Input: dimensioned drawing with shaded views. Units: mm. Origin: part minimum x, y, z. Round coordinates to 2 decimals unless told otherwise and drop trailing zeros. Order: outer loops, then holes, each group sorted by start corner. A loop starts at its lowest first (then second) coordinate and runs counter-clockwise, first axis right, second up. Notation, with made-up numbers: (86, 61) - (104, 61) arc R16 cw to (104, 92) - close; hole circle Ø9 at (72, 69.25). An arc over 180 degrees is marked (long way). One line per item, written item: value. Start each with the question number.
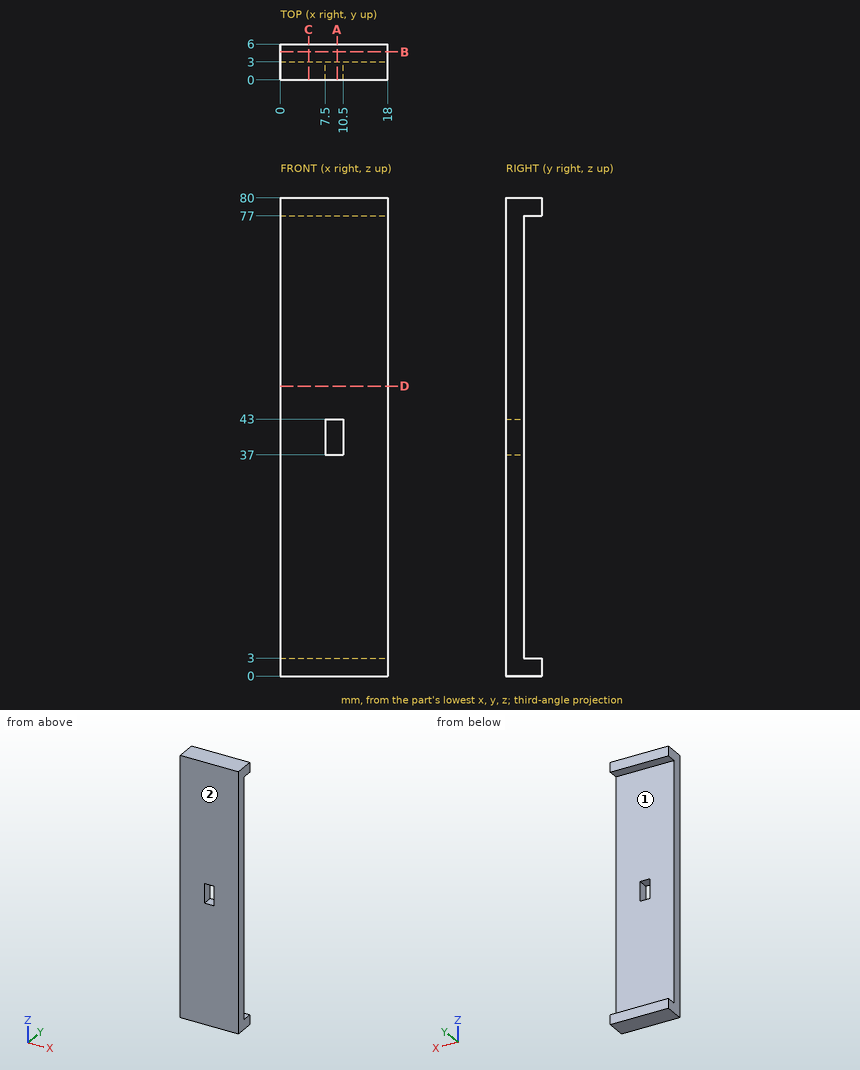
1. Section B-B (y = 4.7). Return the cut outline in (x, z), then the cut area to 3 significant figures.
2. Pull-direction query (Z, two-part tool) for the marked faces 1 and 2; classes: released by +Z, released by -Z, zero draft, split by the parting line, or undercut.
3. Section D-D (z = 48.5). Return the cut outline in (x, y).
4. Section A-A (x = 9.5). Return the cut outline in (y, z), then the cut area to 3 significant figures.
5. Section C-C (x = 4.75). Return the cut outline in (y, z).
6. Line query: line 1 (Z direction, x = 9.5, y = 3.5); line 2 (Y direction, x = 13, z = 22). Output: solid intervals per line, ascending. Write a range as from..to.
7. Pin query (flat end, axial travel): pin 1 (10 mm diameter, centred on x = 12.5, z = 41.5, fed in from +Y). Return the tip coordinate at first contact, or that it passes through.
Solved:
1. outline: (0, 0) - (18, 0) - (18, 3) - (0, 3) - close; (0, 77) - (18, 77) - (18, 80) - (0, 80) - close
1. area: 108 mm²
2. face 1: undercut
2. face 2: zero draft
3. outline: (0, 0) - (18, 0) - (18, 3) - (0, 3) - close
4. outline: (0, 0) - (6, 0) - (6, 3) - (3, 3) - (3, 37) - (0, 37) - close; (0, 43) - (3, 43) - (3, 77) - (6, 77) - (6, 80) - (0, 80) - close
4. area: 240 mm²
5. outline: (0, 0) - (6, 0) - (6, 3) - (3, 3) - (3, 77) - (6, 77) - (6, 80) - (0, 80) - close
6. line 1: z = 0..3, 77..80
6. line 2: y = 0..3
7. pin 1: stops at y = 3
